Design review of the part built by this model. Coordinates are the model's own, in mm. Coordinates: 2 decimals unless noted, no trailing zeros. Write each loop counter-clockwise with the first axis right and the second up, starting at its lowest first coordinate (ties: lowest second). Pieces come first, ordered by that corner, then holes. Notation, with made-up numbers: (15, 67.25) -> (46, 67.25) arc R5 cw to (46, 73.25) -> close; hole circle Ø7 at (29.5, 64.5). An arc over 180 degrees is marked (long way). Return JSON: item names as keys, results as strings. Group by question number.
from build123d import *

# Parameters (mm, degrees)
F0_R     = 1.5
F1_DEPTH = 5
F2_R     = 1
F3_DEPTH = 3
F5_ANGLE = 90
F7_ANGLE = 90


with BuildPart() as f1:
    # F0 (on Top) → F1 (new body)
    with BuildSketch(Plane.XY):
        Polygon((2, 3.5), (-2, 3.5), (-4.020726, 0), (-2, -3.5), (2, -3.5), (4.020726, 0), align=None)
        Circle(F0_R, mode=Mode.SUBTRACT)
    extrude(amount=F1_DEPTH)

    # F2 (on face) → F3 (cut)
    with BuildSketch(Plane.XZ.offset(3.5)):
        with Locations((0, 2.5)):
            Circle(F2_R)
    extrude(amount=-F3_DEPTH, mode=Mode.SUBTRACT)


with BuildPart() as f1_1:
    # F5: moved
    add(f1.part.rotate(Axis((2.035894, 0, 0), (1, 0, 0)), F5_ANGLE))


with BuildPart() as f1_2:
    # F7: moved
    add(f1_1.part.rotate(Axis((0, 0.571142, 0), (0, -1, 0)), F7_ANGLE))


solid = f1_2.part
Q1. For P1, Ø2, axis at x = -2.5, y = -1, coming from the +Z side; P2, Ø3, axis at x = 2.5, y = -2, coming from the -Z side; P3, Ø1.2, axis at y = -2.5, z = 0, coming from the +X side, all flat-tipped, find the tip position at first contact; note any pin that passes through.
Q2. We need section B-B on y = -2.5. Write out the cut boundary in (x, z), plus the area to 3 significant figures.
Q3. Wall thickness on L1, parallel to X at y = -1.35, z = 0; L2, parallel to Z at x = -1, y = -3.55; L3, parallel to Z at x = 0.75, y = -1.3: over which ranges is each line inside the solid? List them lowest first.
Q4. We need section C-C on x = 0.5. Write out the cut boundary in (y, z), plus the area to 3 significant figures.
Q5. We need section D-D on y = -4.4. Write out the cut boundary in (x, z), plus the area to 3 significant figures.
Q6. We need section A-A on z = 0. Write out the cut boundary in (x, y).
Q7. The part is to be moulded in two halves that separate along Y. For faces 1 (the flat face through (0, 0, 2)), 2 (the flat face through (3.5, -1, 0)), 3 (the cylindrical face through (2.326, -2.8, 0.954)), say which applies: +Y half, -Y half, draft (parallel to the pull), parting line (faces both ways), or undercut.
Findings below:
{
 "1": {"P1": "stops at z = 3.15", "P2": "stops at z = -3.44", "P3": "stops at x = -1.37"},
 "2": {"outline": "(-3.5, -2) -> (0, -4.02) -> (3.5, -2) -> (3.5, -1) -> (1.12, -1) arc R1.5 cw (long way) to (1.12, 1) -> (3.5, 1) -> (3.5, 2) -> (0, 4.02) -> (-3.5, 2) -> close", "area": "30.8 mm^2"},
 "3": {"L1": "x = -3.5 to -1.5, 1.5 to 3.5", "L2": "z = -3.44 to -1.12, 1.12 to 3.44", "L3": "z = -3.59 to -1.3, 1.3 to 3.59"},
 "4": {"outline": "(-5, -3.73) -> (0, -3.73) -> (0, -1.41) -> (-5, -1.41) -> close; (-5, 1.41) -> (0, 1.41) -> (0, 3.73) -> (-5, 3.73) -> close", "area": "23.2 mm^2"},
 "5": {"outline": "(-3.5, -2) -> (0, -4.02) -> (3.5, -2) -> (3.5, 2) -> (0, 4.02) -> (-3.5, 2) -> close; hole circle Ø3 at (0, 0)", "area": "35.1 mm^2"},
 "6": {"outline": "(-3.5, -5) -> (-1.5, -5) -> (-1.5, 0) -> (-3.5, 0) -> close; (1.5, -5) -> (3.5, -5) -> (3.5, -3.5) -> (1.5, -3.5) -> close; (1.5, -1.5) -> (3.5, -1.5) -> (3.5, 0) -> (1.5, 0) -> close"},
 "7": {"face 1": "+Y half", "face 2": "draft", "face 3": "undercut"}
}
